Part model, mm, in its own coordinate system. Face numbers are marked on the shaded views. A direction names the side the tool comes from. Round coordinates to 2 decimals unless told otherwise and drop trailing zeros. Write each loop counter-clockwise with the first axis right and the second up, starting at its lowest first coordinate (ties: lowest second). Pieces come first, ordered by that corner, then holes. Notation, with made-up numbers: (49, 13.5) -> (88, 13.5) arc R28 ccw to (88, 49.5) -> close; hole circle Ø4 at (43, 45.5). An arc over 180 degrees is marked (long way). Return JSON: item names as keys, results as strings. Group by question number.
(1) Drop a flat-ended pin along its axis: pin 1 Ø3 at (y, z) = (0, 5) entering from +X. Give the stop position or say it passes through.
(2) Saw through at A-A (y = 0). List the corners of the cut face in (x, z).
(3) Saw through at C-C (x = 0.5). List the corners of the cut face in (y, z).
(4) Mould opens along Y. For the marked faces 3, 4 and 5 say: +Y half, -Y half, draft (parallel to the pull), parting line (faces both ways), or undercut.
(5) Saw through at D-D (z = 5.25). List the corners of the cut face in (x, y), plus the area to 3 significant figures.
(6) Saw through at B-B (z = 7.75). List the corners of the cut face in (x, y).
(7) Drill centre lines: L1, parallel to X at y = 0, z = 8.8; L2, parallel to Z at x = -2.2, y = 0. Where is each one in solid material? Low to high. Write a range as from..to.
(8) Tool access for the marked faces 1 and 2: list every direction of +Z, -Z, +X, -X, +Y, -Y with a clear straight run to the whole face (end or side of a thin tool).
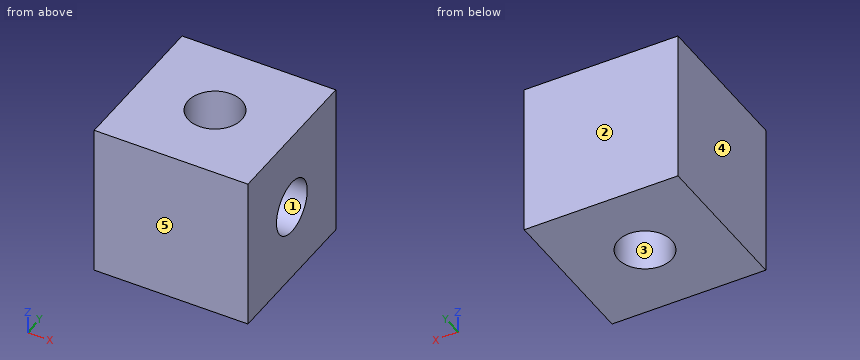
from build123d import *

# Parameters (mm, degrees)
SKETCH1_W           = 10
SKETCH1_H           = 10
SKETCH1_R           = 1.75
BOSS_EXTRUDE1_DEPTH = 10
SKETCH2_R           = 1.75
CUT_EXTRUDE1_DEPTH  = 8


with BuildPart() as part:
    # Sketch1 → Boss-Extrude1 (new body)
    with BuildSketch(Plane.XY):
        Rectangle(SKETCH1_W, SKETCH1_H)
        Circle(SKETCH1_R, mode=Mode.SUBTRACT)
    extrude(amount=BOSS_EXTRUDE1_DEPTH)

    # Sketch2 → Cut-Extrude1 (cut)
    with BuildSketch(Plane(origin=(5, 0, 0), x_dir=(0, 0, -1), z_dir=(1, 0, 0))):
        with Locations((-5, 0)):
            Circle(SKETCH2_R)
    extrude(amount=-CUT_EXTRUDE1_DEPTH, mode=Mode.SUBTRACT)


solid = part.part
Computed values:
{
 "1": {"pin 1": "x = -3"},
 "2": {"outline": "(-5, 0) -> (-1.75, 0) -> (-1.75, 3.25) -> (-3, 3.25) -> (-3, 6.75) -> (-1.75, 6.75) -> (-1.75, 10) -> (-5, 10) -> close; (1.75, 0) -> (5, 0) -> (5, 3.25) -> (1.75, 3.25) -> close; (1.75, 6.75) -> (5, 6.75) -> (5, 10) -> (1.75, 10) -> close"},
 "3": {"outline": "(-5, 0) -> (-1.68, 0) -> (-1.68, 4.5) arc R1.75 cw to (-1.68, 5.5) -> (-1.68, 10) -> (-5, 10) -> close; (1.68, 0) -> (5, 0) -> (5, 10) -> (1.68, 10) -> (1.68, 5.5) arc R1.75 cw to (1.68, 4.5) -> close"},
 "4": {"face 3": "undercut", "face 4": "draft", "face 5": "-Y half"},
 "5": {"outline": "(-5, -5) -> (5, -5) -> (5, -1.73) -> (0.25, -1.73) arc R1.75 cw to (-0.25, -1.73) -> (-3, -1.73) -> (-3, 1.73) -> (-0.25, 1.73) arc R1.75 cw to (0.25, 1.73) -> (5, 1.73) -> (5, 5) -> (-5, 5) -> close", "area": "72.3 mm2"},
 "6": {"outline": "(-5, -5) -> (5, -5) -> (5, 5) -> (-5, 5) -> close; hole circle Ø3.5 at (0, 0)"},
 "7": {"L1": "-5..-1.75, 1.75..5", "L2": "0..3.25, 6.75..10"},
 "8": {"face 1": "+X", "face 2": "+Z, -Z, +X, -X, +Y"}
}
